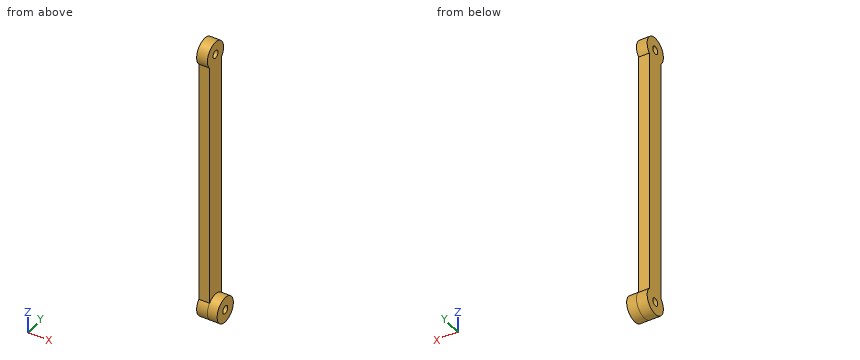
from build123d import *

# Parameters (mm, degrees)
SKETCH1_R           = 2
BOSS_EXTRUDE1_DEPTH = 5.5
SKETCH2_R           = 6.5
SKETCH2_R_2         = 2
BOSS_EXTRUDE3_DEPTH = 5


with BuildPart() as part:
    # Sketch1 → Boss-Extrude1 (new body)
    with BuildSketch(Plane(origin=(0, 0, 0), x_dir=(0, 0, -1), z_dir=(1, 0, 0))):
        with BuildLine():
            Line((4.437059837, 4.75), (130.562940163, 4.75))
            ThreePointArc((130.562940163, 4.75), (141.5, 0), (130.562940163, -4.75))
            Line((130.562940163, -4.75), (4.437059837, -4.75))
            ThreePointArc((4.437059837, -4.75), (-6.5, 0), (4.437059837, 4.75))
        make_face()
        Circle(SKETCH1_R, mode=Mode.SUBTRACT)
        with Locations((135, 0)):
            Circle(SKETCH1_R, mode=Mode.SUBTRACT)
    extrude(amount=BOSS_EXTRUDE1_DEPTH)

    # Sketch2 → Boss-Extrude3 (add)
    with BuildSketch(Plane(origin=(5.5, 0, 0), x_dir=(0, 0, -1), z_dir=(1, 0, 0))):
        with Locations(Location((135, 0, 0), (0, 0, 133.0490798))):
            Circle(SKETCH2_R)
        with Locations((135, 0)):
            Circle(SKETCH2_R_2, mode=Mode.SUBTRACT)
    extrude(amount=BOSS_EXTRUDE3_DEPTH)


solid = part.part
Geometry: final body of the model. Coordinates: model frame, mm. Round coordinates to 2 decimals unless told otherwise and drop trailing zeros. Loops run counter-clockwise (first coordinate to the right, second up) from the corner with the lowest first, then second, coordinate; pieces in that order, holes last. Notation, with made-up numbers: M 80.5,4 L 104.5,4 A19 cw 104.5,37 Z; hole C 10.5,34 d6. An arc over 180 degrees is marked long. Put each result on its own line as item: value. Start each with the question number.
(1) Material intervals for line 1 along Z through (x, y) = (9, 0.25); line 2 along Y through (x, z) = (3.4, 0); line 3 along X through (y, z) = (-1, -39.5), sorted ascending. Write a range as [from, to].
(2) Section query B-B (z = -135). Return loops of the section in (x, y).
(3) Section query D-D (z = 0). Return loops of the section in (x, y).
(4) Contact query for flat-ended pins moving along their axis: pin 1 Ø3 at (x, z) = (2, -65.5) entering from +Y; pin 2 Ø3 at (x, z) = (1.5, -121.5) entering from -Y; pin 3 Ø6 at (x, y) = (8, 3.5) entering from -Z. Output: stop coordinate, or through.
(5) Section query C-C (x = 3.75). Return loops of the section in (y, z).
(6) Section query A-A (y = 0). Return loops of the section in (x, z).
Findings below:
1. line 1: z = [-141.5, -136.98], [-133.02, -128.5]
1. line 2: y = [-6.5, -2], [2, 6.5]
1. line 3: x = [0, 5.5]
2. outline: M 0,-6.5 L 10.5,-6.5 L 10.5,-2 L 0,-2 Z; M 0,2 L 10.5,2 L 10.5,6.5 L 0,6.5 Z
3. outline: M 0,-6.5 L 5.5,-6.5 L 5.5,-2 L 0,-2 Z; M 0,2 L 5.5,2 L 5.5,6.5 L 0,6.5 Z
4. pin 1: stops at y = 4.75
4. pin 2: stops at y = -4.75
4. pin 3: stops at z = -141.48
5. outline: M -4.75,-130.56 A6.5 ccw long 4.75,-130.56 L 4.75,-4.44 A6.5 ccw long -4.75,-4.44 Z; hole C 0,-135 d4; hole C 0,0 d4
6. outline: M 0,-141.5 L 10.5,-141.5 L 10.5,-137 L 0,-137 Z; M 0,-133 L 10.5,-133 L 10.5,-128.5 L 5.5,-128.5 L 5.5,-2 L 0,-2 Z; M 0,2 L 5.5,2 L 5.5,6.5 L 0,6.5 Z
